The listing builds one solid part. Answer for the finished solid, in the listing's coordinates (mm). Face numbers are marked on the shaded views. A direction names the side the tool comes from. Round coordinates to 2 decimals unless told otherwise and drop trailing zeros. Order: outer loops, then holes, each group sorted by start corner. A loop starts at its lowest first (then second) coordinate and runs counter-clockwise, first axis right, second up. Notation, with made-up numbers: (72, -18) -> (118, -18) arc R29 ccw to (118, 20) -> close; hole circle Ø3 at (1.5, -19). An arc over 180 degrees is marked (long way). Answer in a Markdown table with one row per item. Add a question column.
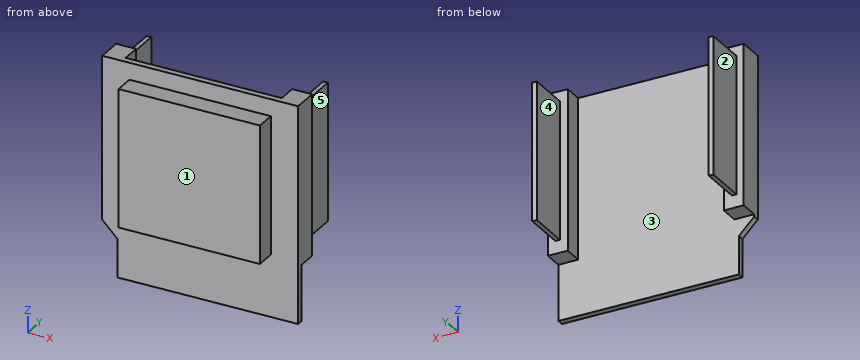
```python
from build123d import *

# Parameters (mm, degrees)
F0_W      = 25.63
F0_H      = 28.3
F1_DEPTH  = 0.85
F2_W      = 9.25
F2_H      = 18
F3_DEPTH  = 2.6
F4_W      = 2
F4_H      = 7
F5_DEPTH  = 25
F6_SIZE   = 1.99999
F7_W      = 2.6
F7_H      = 21
F8_DEPTH  = 2.5
F9_W      = 0.6
F9_H      = 18
F10_DEPTH = 5.5


# Not quite as in the source:
# - a fillet or chamfer is up to 0.001 mm smaller than in the source, because OpenCascade refuses the exact size


with BuildPart() as f1:
    # F0 (on Front) → F1 (new body)
    with BuildSketch(Plane.XZ):
        with Locations((12.815, -14.15)):
            Rectangle(F0_W, F0_H)
    extrude(amount=F1_DEPTH)

    # F2 (on face) → F3 (join)
    with BuildSketch(Plane.XZ.offset(0.85)):
        with Locations((8.19, -11.2)):
            Rectangle(F2_W, F2_H)
        with Locations((17.44, -11.2)):
            Rectangle(F2_W, F2_H)
    extrude(amount=F3_DEPTH)

    # F4 (on face) → F5 (cut)
    with BuildSketch(Plane.XZ.offset(0.85)):
        with Locations((1, -24.8)):
            Rectangle(F4_W, F4_H)
    extrude(amount=-F5_DEPTH, mode=Mode.SUBTRACT)

    # F6 (size 2 in the source; OpenCascade refuses exactly that, so slightly less here)
    f6_edges = [f1.edges().sort_by_distance(p)[0] for p in [
        (2, -0.425, -21.3),
    ]]
    chamfer(f6_edges, length=F6_SIZE)

    # F7 (on face) → F8 (join)
    with BuildSketch(Plane(origin=(0, 0, 0), x_dir=(-1, 0, 0), z_dir=(0, 1, 0))):
        with Locations((-1.3, -10.5)):
            Rectangle(F7_W, F7_H)
        with Locations((-24.33, -10.5)):
            Rectangle(F7_W, F7_H)
    extrude(amount=F8_DEPTH)

    # F9 (on face) → F10 (join)
    with BuildSketch(Plane(origin=(0, 2.5, 0), x_dir=(-1, 0, 0), z_dir=(0, 1, 0))):
        with Locations((-1.2680477372, -10.3143126089)):
            Rectangle(F9_W, F9_H)
        with Locations((-24.3619522628, -10.3143126089)):
            Rectangle(F9_W, F9_H)
    extrude(amount=F10_DEPTH)


solid = f1.part
```
Item 1: Flat-ended cylindrical pins translate along their axes: P1, Ø0.7, axis at x = 1.5, y = 4.5, coming from the -Z side; P2, Ø1, axis at x = 9, y = 1.5, coming from the -Z side; P3, Ø4, axis at y = 4, z = -6.5, coming from the +X side; P4, Ø2, axis at x = 13, y = -2, coming from the -Z side. Find the tip coordinate at first contact, or state that the pin passes through.
Item 2: A tool of negligible diameter and unlimited length cuts with its end or side. For the marked faces 4 and 5, from which of +Z, -Z, +X, -X, +Y, -Y can it reach the whole face along a straight path? Write none if from no direction.
Item 3: The part is cut by section C-C, the plane z = -16.5. Give the vertices of the cut face in (x, y) (3 decimals), and give its area (3 significant figures).
Item 4: Find the intervals of material crossed by probe 1 along X at (y, z) = (7.25, -17.5); probe 2 along Z at (x, y) = (11.25, -1); probe 3 along Y at (x, z) = (20.25, -25), in increasing order. Write a range as [from, to].
Item 5: For a pull along X with two mould halves and no side action, classify the marked faces 1, 2 and 3 as released by +X, released by -X, zero draft, split by the parting line, or undercut.
Item 6: The part is cut by section A-A, the plane y = 1.25. Give the vertices of the cut face in (x, z).
Item 7: The part is cut by section B-B, the plane x = 9.25. Give the vertices of the cut face in (y, z), and give its area (3 significant figures).
Resolved:
| question | item | result |
|---|---|---|
| 1 | P1 | z = -19.31 |
| 1 | P2 | through |
| 1 | P3 | x = 25.63 |
| 1 | P4 | z = -20.2 |
| 2 | face 4 | +Z, -Z, +Y |
| 2 | face 5 | +Z, -Z, +X, +Y |
| 3 | outline | (0, -0.85) -> (3.565, -0.85) -> (3.565, -3.45) -> (22.065, -3.45) -> (22.065, -0.85) -> (25.63, -0.85) -> (25.63, 2.5) -> (24.662, 2.5) -> (24.662, 8) -> (24.062, 8) -> (24.062, 2.5) -> (23.03, 2.5) -> (23.03, 0) -> (2.6, 0) -> (2.6, 2.5) -> (1.568, 2.5) -> (1.568, 8) -> (0.968, 8) -> (0.968, 2.5) -> (0, 2.5) -> close |
| 3 | area | 89.5 mm2 |
| 4 | probe 1 | [0.97, 1.57], [24.06, 24.66] |
| 4 | probe 2 | [-20.2, -2.2] |
| 4 | probe 3 | [-0.85, 0] |
| 5 | face 1 | zero draft |
| 5 | face 2 | released by -X |
| 5 | face 3 | undercut |
| 6 | outline | (0, -21) -> (2.6, -21) -> (2.6, 0) -> (0, 0) -> close; (23.03, -21) -> (25.63, -21) -> (25.63, 0) -> (23.03, 0) -> close |
| 7 | outline | (-3.45, -20.2) -> (-0.85, -20.2) -> (-0.85, -28.3) -> (0, -28.3) -> (0, 0) -> (-0.85, 0) -> (-0.85, -2.2) -> (-3.45, -2.2) -> close |
| 7 | area | 70.9 mm2 |
